The model under review builds one solid part; all positions refer to its coordinate system, in mm. A direction names the side the tool comes from. Coordinates: 2 decimals unless noted, no trailing zeros. Write each loop counter-clockwise with the first axis right and the second up, starting at its lowest first coordinate (ties: lowest second). Pieces come first, ordered by that corner, then holes.
```python
from build123d import *

# Parameters (mm, degrees)
SKETCH1_W           = 6.05
SKETCH1_H           = 20
SKETCH2_W           = 12.1
SKETCH2_H           = 12.1
BOSS_EXTRUDE1_DEPTH = 9.525
SKETCH3_R           = 1.652922186
BOSS_EXTRUDE2_DEPTH = 9.525


with BuildPart() as part:
    # Sketch1 → Revolve1 (revolve)
    with BuildSketch(Plane.XY):
        with Locations((-3.025, 0)):
            Rectangle(SKETCH1_W, SKETCH1_H)
    revolve(axis=Axis((0, 10, 0), (0, -1, 0)))

    # Sketch2 → Boss-Extrude1 (add)
    with BuildSketch(Plane(origin=(0, 10, 0), x_dir=(1, 0, 0), z_dir=(0, 1, 0))):
        Rectangle(SKETCH2_W, SKETCH2_H)
    extrude(amount=BOSS_EXTRUDE1_DEPTH)

    # Sketch3 → Boss-Extrude2 (add)
    with BuildSketch(Plane(origin=(0, 19.525, 0), x_dir=(1, 0, 0), z_dir=(0, 1, 0))):
        Circle(SKETCH3_R)
    extrude(amount=BOSS_EXTRUDE2_DEPTH)


solid = part.part
```
Item 1: For pin 1 (1.5 mm diameter, centred on x = 4.5, z = -5, fed in from +Y) (3 decimals); pin 2 (6 mm diameter, centred on y = 0.5, z = -3.5, fed in from -X), all flat-tipped, find the tip position at first contact; note any pin that passes through.
Solved:
pin 1: stops at y = 19.525
pin 2: stops at x = -6.03
Item 2: To check wall thickness, follow line 1 along Y through (x, z) = (2, -5.25) (3 decimals); line 2 along X through (y, z) = (0.5, -4.5); line 3 along Z through (x, y) = (-0.5, 21). State the ranges of each line that lie inside material, in increasing order.
Solved:
line 1: y = -10 to 19.525
line 2: x = -4.04 to 4.04
line 3: z = -1.58 to 1.58
Item 3: Machinability: for faces 1 (the face through (5, 10, 5)), 2 (the face through (-1.4, 19.525, -1.4)), 3 (the face through (-5, 10, -5)), 4 (the face through (5, 10, -5)), which of the approach directions +Z, -Z, +X, -X, +Y, -Y give a long, thin tool a straight path to every point of the face, cutting with its end or side? Answer none if there is none.
Solved:
face 1: +Z, +X, -Y
face 2: +Y
face 3: -Z, -X, -Y
face 4: -Z, +X, -Y
Item 4: Take a section at D-D, the plane x = -0.5. Write out the cut boundary in (y, z) (3 decimals), plus the area to 3 significant figures.
Solved:
outline: (-10, -6.029) - (10, -6.029) - (10, -6.05) - (19.525, -6.05) - (19.525, -1.575) - (29.05, -1.575) - (29.05, 1.575) - (19.525, 1.575) - (19.525, 6.05) - (10, 6.05) - (10, 6.029) - (-10, 6.029) - close
area: 386 mm2
Item 5: Take a section at B-B, the plane y = 23. Write out the cut boundary in (x, z).
Solved:
outline: circle Ø3.31 at (0, 0)
Item 6: Take a section at A-A, the plane x = 4. Write out the cut boundary in (y, z) (3 decimals), plus the area to 3 significant figures.
Solved:
outline: (-10, -4.539) - (10, -4.539) - (10, -6.05) - (19.525, -6.05) - (19.525, 6.05) - (10, 6.05) - (10, 4.539) - (-10, 4.539) - close
area: 297 mm2
Item 7: Take a section at C-C, the plane z = 3. Write out the cut boundary in (x, y) (3 decimals).
Solved:
outline: (-6.05, 10) - (-5.254, 10) - (-5.254, -10) - (5.254, -10) - (5.254, 10) - (6.05, 10) - (6.05, 19.525) - (-6.05, 19.525) - close
